```python
from build123d import *

# Parameters (mm, degrees)
SKETCH1_W           = 125
SKETCH1_H           = 62
SKETCH1_R           = 7.5
BOSS_EXTRUDE1_DEPTH = 12
BOSS_EXTRUDE3_DEPTH = 125
SKETCH7_W           = 12
SKETCH7_H           = 74
BOSS_EXTRUDE6_DEPTH = 15
SKETCH8_W           = 12.503423745
SKETCH8_H           = 50
BOSS_EXTRUDE7_DEPTH = 62
CUT_EXTRUDE1_DEPTH  = 62
FILLET1_R           = 10
FILLET2_R           = 10
SKETCH10_R          = 7.5
CUT_EXTRUDE2_DEPTH  = 12
SKETCH11_R          = 6
CUT_EXTRUDE3_DEPTH  = 12


with BuildPart() as part:
    # Sketch1 → Boss-Extrude1 (new body)
    with BuildSketch(Plane(origin=(0, 0, 0), x_dir=(1, 0, 0), z_dir=(0, 1, 0))):
        with Locations((62.5, 31)):
            Rectangle(SKETCH1_W, SKETCH1_H)
        with Locations(Location((15, 15, 0), (0, 0, 270))):
            Circle(SKETCH1_R, mode=Mode.SUBTRACT)
        with Locations(Location((110, 47, 0), (0, 0, 270))):
            Circle(SKETCH1_R, mode=Mode.SUBTRACT)
    extrude(amount=BOSS_EXTRUDE1_DEPTH)

    # Sketch2 → Boss-Extrude3 (add)
    with BuildSketch(Plane(origin=(125, 0, 0), x_dir=(0, 0, -1), z_dir=(1, 0, 0))):
        Polygon((62, 0), (62, -12), (74, -12), (74, 62), (62, 62), (62, 12), (0, 12), (0, 0), align=None)
    extrude(amount=-BOSS_EXTRUDE3_DEPTH)

    # Sketch7 → Boss-Extrude6 (add)
    with BuildSketch(Plane(origin=(0, 0, -74), x_dir=(-1, 0, 0), z_dir=(0, 0, -1))):
        with Locations((-76.226215006, 25)):
            Rectangle(SKETCH7_W, SKETCH7_H)
        with Locations((-44.226215006, 25)):
            Rectangle(SKETCH7_W, SKETCH7_H)
    extrude(amount=BOSS_EXTRUDE6_DEPTH)

    # Sketch8 → Boss-Extrude7 (add)
    with BuildSketch(Plane.XY.offset(-62)):
        with Locations((60.823295538, 37)):
            Rectangle(SKETCH8_W, SKETCH8_H)
    extrude(amount=BOSS_EXTRUDE7_DEPTH)

    # Sketch9 → Cut-Extrude1 (cut)
    with BuildSketch(Plane(origin=(67.07500741, 0, 0), x_dir=(0, 0, -1), z_dir=(1, 0, 0))):
        Polygon((0, 12), (62, 62), (0, 62), align=None)
    extrude(amount=-CUT_EXTRUDE1_DEPTH, mode=Mode.SUBTRACT)

    # Fillet1
    fillet1_edges = [part.edges().sort_by_distance(p)[0] for p in [
        (125, 62, -68),
    ]]
    fillet(fillet1_edges, radius=FILLET1_R)

    # Fillet2
    fillet2_edges = [part.edges().sort_by_distance(p)[0] for p in [
        (0, 62, -68),
    ]]
    fillet(fillet2_edges, radius=FILLET2_R)

    # Sketch10 → Cut-Extrude2 (cut)
    with BuildSketch(Plane(origin=(0, 12, 0), x_dir=(1, 0, 0), z_dir=(0, 1, 0))):
        with Locations(Location((15, 15, 0), (0, 0, 270))):
            Circle(SKETCH10_R)
        with Locations(Location((110, 47, 0), (0, 0, 270))):
            Circle(SKETCH10_R)
    extrude(amount=-CUT_EXTRUDE2_DEPTH, mode=Mode.SUBTRACT)

    # Sketch11 → Cut-Extrude3 (cut)
    with BuildSketch(Plane.XY.offset(-62)):
        with Locations((105, 42)):
            Circle(SKETCH11_R)
        with Locations((20, 42)):
            Circle(SKETCH11_R)
    extrude(amount=-CUT_EXTRUDE3_DEPTH, mode=Mode.SUBTRACT)


solid = part.part
```
For this review, take the finished solid that the model builds, in its own axes (mm). A direction names the side the tool comes from. Round coordinates to 2 decimals unless told otherwise and drop trailing zeros. Write each loop counter-clockwise with the first axis right and the second up, starting at its lowest first coordinate (ties: lowest second). Pieces come first, ordered by that corner, then holes. Notation, with made-up numbers: (81.5, 35) - (134.5, 35) arc R24 cw to (134.5, 52) - close; hole circle Ø11 at (6, 54). An arc over 180 degrees is marked (long way). Answer as a JSON object with one key per item and string values.
1. Tool access review of faces 4 (the face through (104, 24, -74)), 5 (the face through (70.226, 24, -81)), 6 (the face through (38.226, 24, -81)), 7 (the face through (96, 37, -62)), 8 (the face through (28, 37, -62)): name each direction out of +Z, -Z, +X, -X, +Y, -Y from which nothing blocks a thin tool from reaching the whole face with its end or side.
Response values:
{"face 4": "-Z, +X, +Y, -Y", "face 5": "-Z, +Y, -Y", "face 6": "-Z, -X, +Y, -Y", "face 7": "+Z, +X, +Y", "face 8": "+Z, -X, +Y"}
2. We need section C-C on z = -49. Give the boundary of the cut face in (x, y) (3 decimals).
Response values:
{"outline": "(0, 0) - (102.772, 0) - (102.772, 12) - (67.075, 12) - (67.075, 51.516) - (54.572, 51.516) - (54.572, 12) - (0, 12) - close; (117.228, 0) - (125, 0) - (125, 12) - (117.228, 12) - close"}
3. Draft analysis for pull direction X (two halves, no side actions). For faces 1 (the face through (60, 24, -74)), 2 (the face through (3.01, 59.15, -67.92)), 3 (the face through (67.075, 31, -38)), state which applies: +X half, -X half, draft (parallel to the pull), parting line (faces both ways), or undercut.
Response values:
{"face 1": "undercut", "face 2": "-X half", "face 3": "+X half"}
4. For pin 1 Ø25 at (y, z) = (40, -44) entering from -X; pin 2 Ø16.5 at (y, z) = (11, -84.5) entering from +X; pin 3 Ø6 at (x, z) = (43, -34.5) entering from -Y, all flat-tipped, find the tip position at first contact; note any pin that passes through.
Response values:
{"pin 1": "stops at x = 54.57", "pin 2": "stops at x = 82.23", "pin 3": "stops at y = 0"}
5. We need section A-A on x = 29. Give the boundary of the cut face in (y, z), then the cut area to 3 significant figures.
Response values:
{"outline": "(-12, -74) - (62, -74) - (62, -62) - (12, -62) - (12, 0) - (0, 0) - (0, -62) - (-12, -62) - close", "area": "1,630 mm2"}
6. We need section D-D on y = 5. Give the boundary of the cut face in (x, z), then the cut area to 3 significant figures.
Response values:
{"outline": "(0, -74) - (38.23, -74) - (38.23, -89) - (50.23, -89) - (50.23, -74) - (70.23, -74) - (70.23, -89) - (82.23, -89) - (82.23, -74) - (125, -74) - (125, 0) - (0, 0) - close; hole circle Ø15 at (15, -15); hole circle Ø15 at (110, -47)", "area": "9,260 mm2"}
7. To check wall thickness, follow line 1 along X through (y, z) = (5.25, -47); line 2 along Y through (x, z) = (20, -64.5); line 3 along X through (y, z) = (57.5, -56.5) (3 decimals). State the ranges of each line that lie inside material, in increasing order.
Response values:
{"line 1": "x = 0 to 102.5, 117.5 to 125", "line 2": "y = -12 to 36, 48 to 62", "line 3": "x = 54.572 to 67.075"}
8. We need section B-B on y = 49.5. Give the boundary of the cut face in (x, z) (3 decimals).
Response values:
{"outline": "(0, -74) - (38.226, -74) - (38.226, -89) - (50.226, -89) - (50.226, -74) - (70.226, -74) - (70.226, -89) - (82.226, -89) - (82.226, -74) - (125, -74) - (125, -62) - (67.075, -62) - (67.075, -46.5) - (54.572, -46.5) - (54.572, -62) - (0, -62) - close"}
